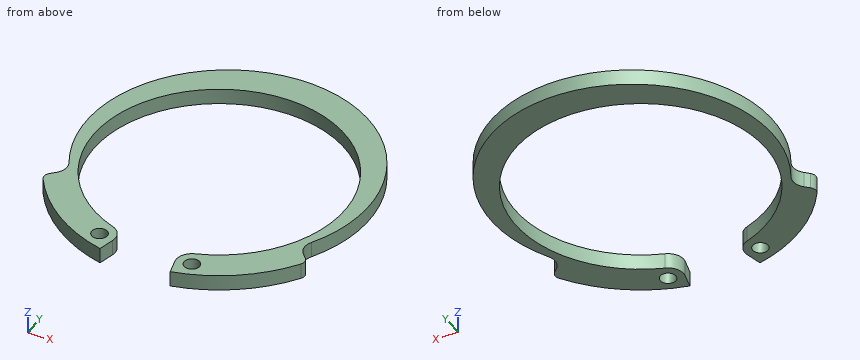
from build123d import *

# Parameters (mm, degrees)
SKETCH1_R           = 0.5
BOSS_EXTRUDE1_DEPTH = 1


with BuildPart() as part:
    # Sketch1 → Boss-Extrude1 (new body)
    with BuildSketch(Plane.XY):
        with BuildLine():
            Line((-8.036806523, -5.559320723), (-8.311889028, -5.834403228))
            ThreePointArc((-8.311889028, -5.834403228), (-8.455641966, -6.136125974), (-8.377195408, -6.461006967))
            ThreePointArc((-8.377195408, -6.461006967), (-5.735345972, -9.191813388), (-2.265503441, -10.739994567))
            Line((-2.265503441, -10.739994567), (-2.032287486, -9.737337896))
            ThreePointArc((-2.032287486, -9.737337896), (-2.116763903, -9.016352811), (-2.666666667, -8.542472333))
            ThreePointArc((-2.666666667, -8.542472333), (0, 7), (2.666666667, -8.542472333))
            ThreePointArc((2.666666667, -8.542472333), (2.116763903, -9.016352811), (2.032287486, -9.737337896))
            Line((2.032287486, -9.737337896), (2.291840404, -10.733831084))
            ThreePointArc((2.291840404, -10.733831084), (5.746419561, -9.184049256), (8.377195408, -6.461006967))
            ThreePointArc((8.377195408, -6.461006967), (8.455641966, -6.136125974), (8.311889028, -5.834403228))
            Line((8.311889028, -5.834403228), (8.036806523, -5.559320723))
            ThreePointArc((8.036806523, -5.559320723), (7.753612497, -4.991153897), (7.869521974, -4.366992547))
            ThreePointArc((7.869521974, -4.366992547), (0, 9), (-7.869521974, -4.366992547))
            ThreePointArc((-7.869521974, -4.366992547), (-7.753612497, -4.991153897), (-8.036806523, -5.559320723))
        make_face()
        with Locations((-3, -9.485281374)):
            Circle(SKETCH1_R, mode=Mode.SUBTRACT)
        with Locations((3, -9.485281374)):
            Circle(SKETCH1_R, mode=Mode.SUBTRACT)
    extrude(amount=BOSS_EXTRUDE1_DEPTH)


solid = part.part
CAD build for the part. Positions are in the model's coordinates, mm. Round coordinates to 2 decimals unless told otherwise and drop trailing zeros. Loops run counter-clockwise (first coordinate to the right, second up) from the corner with the lowest first, then second, coordinate; pieces in that order, holes last.
(1) Cut at A-A (y = -1). Give the cut face in (x, z).
(2) Cut at C-C (z = 0.2). Give the cut face in (x, y).
(3) Cut at D-D (x = 3). Give the cut face in (y, z).
(4) Cut at B-B (x = -4.5). Give the cut face in (y, z), plus the area to 3 significant figures.
(5) Wall check: line 1 along Y through (x, z) = (3, 0.55); line 2 along X through (y, z) = (3.5, 0.3); line 3 along X through (y, z) = (-9.5, 0.3). Give the ranges that are in metal, low to high.
Findings below:
1. outline: (-8.94, 0) - (-8, 0) - (-8, 1) - (-8.94, 1) - close; (8, 0) - (8.94, 0) - (8.94, 1) - (8, 1) - close
2. outline: (-8.38, -6.46) arc R10 ccw to (-2.27, -10.74) - (-2.03, -9.74) arc R1 ccw to (-2.67, -8.54) arc R8 cw (long way) to (2.67, -8.54) arc R1 ccw to (2.03, -9.74) - (2.29, -10.73) arc R10 ccw to (8.38, -6.46) arc R0.5 ccw to (8.31, -5.83) - (8.04, -5.56) arc R1 cw to (7.87, -4.37) arc R9 ccw (long way) to (-7.87, -4.37) arc R1 cw to (-8.04, -5.56) - (-8.31, -5.83) arc R0.5 ccw to start; hole circle Ø1 at (-3, -9.49); hole circle Ø1 at (3, -9.49)
3. outline: (-10.54, 0) - (-9.99, 0) - (-9.99, 1) - (-10.54, 1) - close; (-8.99, 0) - (-8.42, 0) - (-8.42, 1) - (-8.99, 1) - close; (6.42, 0) - (8.49, 0) - (8.49, 1) - (6.42, 1) - close
4. outline: (-9.93, 0) - (-7.61, 0) - (-7.61, 1) - (-9.93, 1) - close; (5.61, 0) - (7.79, 0) - (7.79, 1) - (5.61, 1) - close
4. area: 4.50 mm2
5. line 1: y = -10.54 to -9.99, -8.99 to -8.42, 6.42 to 8.49
5. line 2: x = -8.29 to -6.61, 6.61 to 8.29
5. line 3: x = -5.27 to -3.5, -2.5 to -2, 2 to 2.5, 3.5 to 5.27
